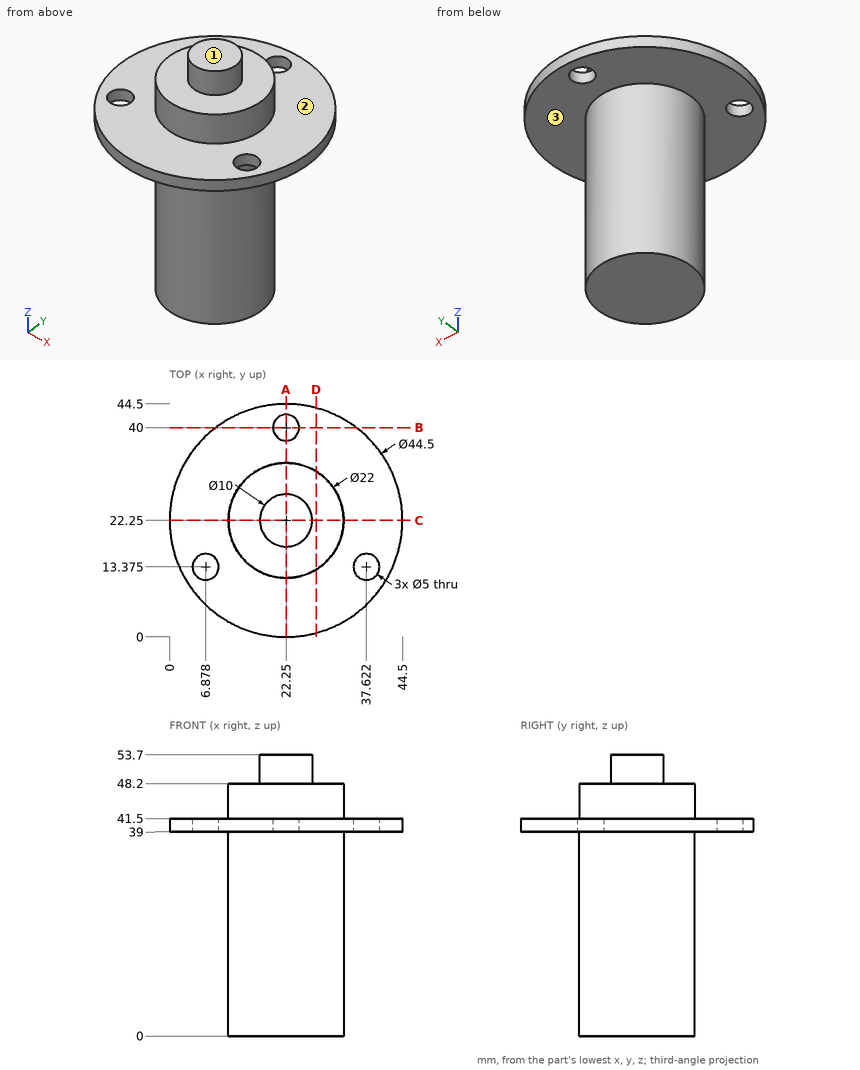
Study the drawing (mm; zero at the part's minimum x, y, z) and answer. A direction names the side the tool comes from. Round coordinates to 2 decimals unless told otherwise and drop trailing zeros. Write each loop counter-clockwise with the first axis right and the second up, starting at its lowest first coordinate (ties: lowest second). Pieces come first, ordered by that corner, then holes. Notation, with made-up numbers: (0, 13.5) - (29, 13.5) arc R21 cw to (29, 41.5) - close; hole circle Ø9 at (-36, 69.25). An arc over 180 degrees is marked (long way). Use a Markdown table: item, result. Add a question column.
1. A tool of negligible diameter and unlimited length cuts with its end or side. For the marked faces 1, 2 and 3, from which of +Z, -Z, +X, -X, +Y, -Y can it reach the whole face along a straight path? Write none if from no direction.
2. The part is cut by section C-C (y = 22.25). Write down the section's boundary in (x, z), and give its area (3 significant figures).
3. Flat-ended cylindrical pins translate along their axes: P1, Ø5, axis at y = 15.5, z = 47.5, coming from the -X side; P2, Ø2, axis at y = 13, z = 11.5, coming from the +X side; P3, Ø10, axis at x = 30, z = 21.5, coming from the -Y side; P4, Ø13.5, axis at x = 13.5, y = 18, coming from the +Z side. Find the tip coordinate at first contact, or state that the pin passes through.
4. The part is cut by section B-B (y = 40). Write down the section's boundary in (x, z), and give its area (3 significant figures).
5. The part is cut by section A-A (x = 22.25). Write down the section's boundary in (y, z), and give its area (3 significant figures).
6. Consider line 1 (Y direction, x = 22.25, z = 40.6); line 2 (Z direction, x = 17.5, y = 33.5); line 3 (Y direction, x = 25.5, z = 40.5). Determine where each line is inside the solid, lowest interval first.
7. The part is cut by section D-D (x = 28). Write down the section's boundary in (y, z), and give its area (3 significant figures).
Reported:
| question | item | result |
|---|---|---|
| 1 | face 1 | +Z, +X, -X, +Y, -Y |
| 1 | face 2 | +Z |
| 1 | face 3 | -Z |
| 2 | outline | (0, 39) - (11.25, 39) - (11.25, 0) - (33.25, 0) - (33.25, 39) - (44.5, 39) - (44.5, 41.5) - (33.25, 41.5) - (33.25, 48.2) - (27.25, 48.2) - (27.25, 53.7) - (17.25, 53.7) - (17.25, 48.2) - (11.25, 48.2) - (11.25, 41.5) - (0, 41.5) - close |
| 2 | area | 1,170 mm^2 |
| 3 | P1 | x = 12.1 |
| 3 | P2 | x = 29.53 |
| 3 | P3 | y = 11.6 |
| 3 | P4 | z = 53.7 |
| 4 | outline | (8.83, 39) - (19.75, 39) - (19.75, 41.5) - (8.83, 41.5) - close; (24.75, 39) - (35.67, 39) - (35.67, 41.5) - (24.75, 41.5) - close |
| 4 | area | 54.6 mm^2 |
| 5 | outline | (0, 39) - (11.25, 39) - (11.25, 0) - (33.25, 0) - (33.25, 39) - (37.5, 39) - (37.5, 41.5) - (33.25, 41.5) - (33.25, 48.2) - (27.25, 48.2) - (27.25, 53.7) - (17.25, 53.7) - (17.25, 48.2) - (11.25, 48.2) - (11.25, 41.5) - (0, 41.5) - close; (42.5, 39) - (44.5, 39) - (44.5, 41.5) - (42.5, 41.5) - close |
| 5 | area | 1,160 mm^2 |
| 6 | line 1 | 0 to 37.5, 42.5 to 44.5 |
| 6 | line 2 | 39 to 41.5 |
| 6 | line 3 | 0.24 to 44.26 |
| 7 | outline | (0.76, 39) - (12.87, 39) - (12.87, 0) - (31.63, 0) - (31.63, 39) - (43.74, 39) - (43.74, 41.5) - (31.63, 41.5) - (31.63, 48.2) - (12.87, 48.2) - (12.87, 41.5) - (0.76, 41.5) - close |
| 7 | area | 965 mm^2 |
